Check sheet for the drawn part. Datum: minimum x, y, z corner. Units: mm. A direction names the side the tool comes from. Round coordinates to 2 decimals unless told otherwise and drop trailing zeros. Write each loop counter-clockwise with the first axis right and the second up, starting at its lowest first coordinate (ties: lowest second). Pieces come first, ordered by that corner, then holes. Notation, with made-up numbers: (24, -15) -> (50, -15) arc R33 cw to (50, 20) -> close; hole circle Ø4 at (-4, 85). An arc over 180 degrees is marked (long way). One line per item, written item: value.
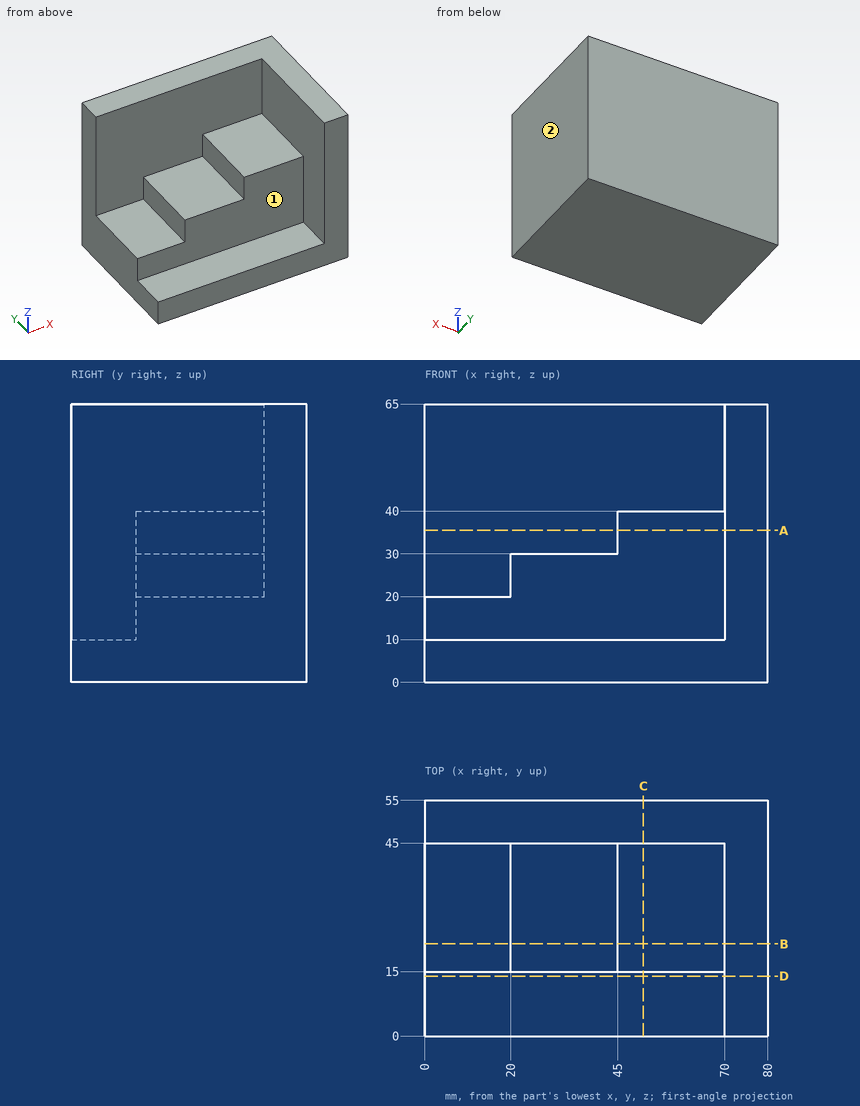
Item 1: Sectioned sample at A-A on z = 35.5. Enter the section's corners in (x, y).
Answer:
outline: (0, 45) -> (45, 45) -> (45, 15) -> (70, 15) -> (70, 0) -> (80, 0) -> (80, 55) -> (0, 55) -> close
Item 2: Sectioned sample at D-D on y = 14. Enter the section's corners in (x, z), and give its area (3 significant figures).
Answer:
outline: (0, 0) -> (80, 0) -> (80, 65) -> (70, 65) -> (70, 10) -> (0, 10) -> close
area: 1,350 mm^2
Item 3: Sectioned sample at C-C on x = 51. Enter the section's corners in (y, z), and give its area (3 significant figures).
Answer:
outline: (0, 0) -> (55, 0) -> (55, 65) -> (45, 65) -> (45, 40) -> (15, 40) -> (15, 10) -> (0, 10) -> close
area: 2,000 mm^2
Item 4: Tool access check on the marked faces 1 and 2. Record the directions out of +Z, -Z, +X, -X, +Y, -Y that give a thin tool (end or side, any length) a straight path to the whole face; none if there is none.
Answer:
face 1: +Z, -X, -Y
face 2: +Z, -Z, +X, +Y, -Y
Item 5: Thickness scan on line 1 (Z direction, x = 14, y = 23.5); line 2 (Z direction, x = 39.5, y = 44.5); line 3 (Y direction, x = 13.5, z = 39). Record the ranges inside material, lowest first.
Answer:
line 1: z = 0 to 20
line 2: z = 0 to 30
line 3: y = 45 to 55
Item 6: Depth check by flat-ended pin: P1, Ø2, axis at x = 15, y = 16.5, coming from the +Z side; P2, Ø11, axis at y = 25, z = 36.5, coming from the -X side; P3, Ø10, axis at x = 29.5, z = 22.5, coming from the -Y side. Enter the tip coordinate at first touch or a pass-through.
Answer:
P1: stops at z = 20
P2: stops at x = 45
P3: stops at y = 15
Item 7: Sectioned sample at B-B on y = 21.5. Enter the section's corners in (x, z).
Answer:
outline: (0, 0) -> (80, 0) -> (80, 65) -> (70, 65) -> (70, 40) -> (45, 40) -> (45, 30) -> (20, 30) -> (20, 20) -> (0, 20) -> close
